The listing builds one solid part. Answer for the finished solid, in the listing's coordinates (mm). A direction names the side the tool comes from. Coordinates: 2 decimals unless noted, no trailing zeros. Write each loop counter-clockwise with the first axis right and the second up, starting at its lowest first coordinate (ties: lowest second). Pieces come first, ordered by that corner, then holes.
from build123d import *

# Parameters (mm, degrees)
SKETCH1_R                = 29.95
BOSS_EXTRUDE1_DEPTH      = 3
FILLET1_R                = 0.5
BOSS_EXTRUDE2_DEPTH      = 8
BOSS_EXTRUDE2_DEPTH_BACK = 17
SKETCH3_R                = 6
CUT_EXTRUDE2_DEPTH       = 14.3
CUT_EXTRUDE4_START       = -14.3
CUT_EXTRUDE4_DEPTH       = 9
SKETCH7_R                = 1.0925
BOSS_EXTRUDE3_DEPTH      = 4
BOSS_EXTRUDE4_DEPTH      = 2


with BuildPart() as part:
    # Sketch1 → Boss-Extrude1 (new body)
    with BuildSketch(Plane(origin=(0, 0, 0), x_dir=(1, 0, 0), z_dir=(0, 1, 0))):
        with Locations(Location((0, 0, 0), (0, 0, 270))):
            Circle(SKETCH1_R)
    extrude(amount=BOSS_EXTRUDE1_DEPTH)

    # Fillet1
    fillet1_edges = [part.edges().sort_by_distance(p)[0] for p in [
        (0, 3, -29.95),
    ]]
    fillet(fillet1_edges, radius=FILLET1_R)

    # Sketch3 → Boss-Extrude2 (add, two sides: drawn at the far end of the back side and taken through both)
    with BuildSketch(Plane.XY.offset(-BOSS_EXTRUDE2_DEPTH_BACK)):
        with BuildLine():
            ThreePointArc((22.319611022, 17.326801635), (25.571028156, 35.421781232), (7.476048559, 38.673198365))
            Line((7.476048559, 38.673198365), (-15.351755113, 22.799515608))
            ThreePointArc((-15.351755113, 22.799515608), (-19.451327013, 18.1478139), (-20.929973881, 12.126317243))
            Line((-20.929973881, 12.126317243), (-20.929973881, 3))
            Line((-20.929973881, 3), (9.161240081, 3))
            Line((9.161240081, 3), (9.161240081, 3.233006236))
            ThreePointArc((9.161240081, 3.233006236), (10.350199335, 7.962230378), (13.634352277, 11.566883557))
            Line((13.634352277, 11.566883557), (22.319611022, 17.326801635))
        make_face()
        with Locations((14.897829791, 28)):
            Circle(SKETCH3_R, mode=Mode.SUBTRACT)
    extrude(amount=BOSS_EXTRUDE2_DEPTH + BOSS_EXTRUDE2_DEPTH_BACK)

    # Sketch5 → Cut-Extrude2 (cut)
    with BuildSketch(Plane(origin=(0, 0, -17), x_dir=(-1, 0, 0), z_dir=(0, 0, -1))):
        with BuildLine():
            Line((-8.626514029, 37.037178687), (14.430028566, 21.037178687))
            ThreePointArc((14.430028566, 21.037178687), (17.905108892, 17.099780712), (19.158712805, 12))
            Line((19.158712805, 12), (19.158712805, 5.262193484))
            Line((19.158712805, 5.262193484), (-7.161240081, 5.262193484))
            Line((-7.161240081, 5.262193484), (-7.161240081, 5.56341477))
            ThreePointArc((-7.161240081, 5.56341477), (-8.137033641, 9.392321128), (-10.826371055, 12.287171944))
            Line((-10.826371055, 12.287171944), (-20.858274701, 18.754833886))
            ThreePointArc((-20.858274701, 18.754833886), (-24.040323598, 34.116764421), (-8.626514029, 37.037178687))
        make_face()
    extrude(amount=-CUT_EXTRUDE2_DEPTH, mode=Mode.SUBTRACT)

    # Sketch4 → Cut-Extrude4 (cut)
    with BuildSketch(Plane(origin=(0, 0, -17), x_dir=(-1, 0, 0), z_dir=(0, 0, -1)).offset(CUT_EXTRUDE4_START)):
        Polygon((-23.261597646, 26.588590728), (-4.523766462, 13.250911675), (2.435022609, 23.027171423), (-16.302808575, 36.364850476), align=None)
    extrude(amount=-CUT_EXTRUDE4_DEPTH, mode=Mode.SUBTRACT)

    # Sketch7 → Boss-Extrude3 (add)
    with BuildSketch(Plane(origin=(0, 0, -2.7), x_dir=(-1, 0, 0), z_dir=(0, 0, -1))):
        with Locations((-21.488975125, 32.691609194)):
            Circle(SKETCH7_R)
        with Locations((0.684110702, 16.95524562)):
            Circle(SKETCH7_R)
    extrude(amount=BOSS_EXTRUDE3_DEPTH)

    # Sketch8 → Boss-Extrude4 (add)
    with BuildSketch(Plane.XZ):
        with BuildLine():
            Line((4.419624532, 5.457754962), (-15.163378573, 4.241831176))
            ThreePointArc((-15.163378573, 4.241831176), (-19.147983311, 0.130911389), (-15.424074318, -4.217564002))
            Line((-15.424074318, -4.217564002), (-14.905016784, -4.249997039))
            Line((-14.905016784, -4.249997039), (4.41534389, -5.457219623))
            Line((4.41534389, -5.457219623), (5.1, -5.5))
            ThreePointArc((5.1, -5.5), (10.6, 0), (5.1, 5.5))
            Line((5.1, 5.5), (4.419624532, 5.457754962))
        make_face()
        with BuildLine():
            Line((-14.9, 2.25), (4.880474733, 3.493108738))
            ThreePointArc((4.880474733, 3.493108738), (8.6, 0), (4.880474733, -3.493108738))
            Line((4.880474733, -3.493108738), (-14.9, -2.25))
            ThreePointArc((-14.9, -2.25), (-17.15, 0), (-14.9, 2.25))
        make_face(mode=Mode.SUBTRACT)
    extrude(amount=BOSS_EXTRUDE4_DEPTH)


solid = part.part
1. Section A-A on y = 28 is taken. Give the vertices of the cut face in (x, z).
Results found:
outline: (-7.87, -17) - (-4.4, -17) - (-4.4, -2.7) - (4.55, -2.7) - (4.55, 6.3) - (8.9, 6.3) - (8.9, 8) - (-7.87, 8) - close; (20.9, 6.3) - (22.26, 6.3) - (22.26, -2.7) - (25.9, -2.7) - (25.9, -17) - (27.9, -17) - (27.9, 8) - (20.9, 8) - close
2. Section C-C on y = 4 is taken. Give the vertices of the cut face in (x, z).
Results found:
outline: (-20.93, -17) - (9.19, -17) - (9.19, 8) - (-20.93, 8) - close
3. For a pull along X with two mould halves and no side action, classify faces 6 (the cylindrical face through (-19.144, -0.986, 0.219)), 7 (the flat face through (-4.87, -0.99, -2.88)), 8 (the flat face through (-6, 28, -17)) as pulls with the +X half, pulls with the -X half, needs draft (parallel to the pull), parting line crosses it, or undercut.
Results found:
face 6: pulls with the -X half
face 7: undercut
face 8: needs draft
4. Find the intervals of material crossed by L1, parallel to Z at x = -9.5, y = 13; L2, parallel to Y at x = 13.5, z = -12.5; L3, parallel to Z at x = 26, y = 26.5, in increasing order.
Results found:
L1: z = -2.7 to 8
L2: y = 0 to 3, 11.48 to 14.01, 38.91 to 40.92
L3: z = -17 to 8
5. A tool of negligible diameter and unlimited length cuts with its end or side. For faces 1 (the cylindrical face through (-17.15, -0.99, -0.05)), 2 (the flat face through (-20.93, 8, -5)), 3 (the flat face through (17.92, 14.41, -4.68)), 4 (the cylindrical face through (-17.87, 17.17, -9.95)), 5 (the cylindrical face through (12.602, 33.544, 7.381)), from which of +Z, -Z, +X, -X, +Y, -Y can it reach the whole face along a straight path? Write none if from no direction.
Results found:
face 1: -Y
face 2: +Z, -Z, -X, +Y
face 3: +Z, -Z, +X
face 4: -Z
face 5: +Z, -Z
6. Section B-B on y = 10.5 is taken. Give the vertices of the cut face in (x, z).
Results found:
outline: (-20.93, -17) - (-19.16, -17) - (-19.16, -2.7) - (8.87, -2.7) - (8.87, -17) - (12.29, -17) - (12.29, 8) - (-20.93, 8) - close
7. Flat-ended cylindrical pins translate along their axes: P1, Ø4, axis at x = 20, y = 30, coming from the +Z side; P2, Ø12, axis at x = -6.5, z = -18.5, coming from the -Y side; P3, Ø1.4, axis at x = 17, y = 33.5, coming from the -Z side. Find the tip coordinate at first contact, or state that the pin passes through.
Results found:
P1: stops at z = 8
P2: stops at y = 0
P3: stops at z = 6.3
